Part model, mm, in its own coordinate system. Face numbers are marked on the shaded views. A direction names the side the tool comes from. Coordinates: 2 decimals unless noted, no trailing zeros. Loops run counter-clockwise (first coordinate to the right, second up) from the corner with the lowest first, then second, coordinate; pieces in that order, holes last. Notation, with made-up numbers: M 80,-28.75 L 96,-28.75 A8 ccw 96,-17.75 Z; hole C 26.25,72.5 d6. An arc over 180 degrees is marked long. Use a Markdown table: item, result. Add a question column.
1) Band-saw the part on D-D (x = 3). List the corners of the cut face in (y, z).
2) Band-saw the part on B-B (y = 1.75). List the corners of the cut face in (x, z), plus the area to 3 significant figures.
3) Tool access for the marked faces 4, 5 and 6: list every direction of +Z, -Z, +X, -X, +Y, -Y with a clear straight run to the whole face (end or side of a thin tool).
4) Band-saw the part on A-A (z = -3.5). List the corners of the cut face in (x, y), plus the area to 3 significant figures.
5) Wall check: probe 1 along Z at (x, y) = (2, 0.55); probe 2 along Z at (x, y) = (3, 2.4); probe 3 along X at (y, z) = (2.05, 3). Give the ranges that are in metal, low to high. Write a range as from..to.
6) Pull direction X, two halves, no side cores. Call the marked faces 1, 2 and 3: released by +X, released by -X, zero draft, split by the parting line, or undercut.
7) Pin check, flat tips, straight feed: pin 1 Ø10.5 at (x, z) = (0, 0) entering from +Y; pin 2 Ø0.9 at (x, y) = (17.5, 2) entering from +Z; pin 3 Ø0.9 at (y, z) = (2, -17) entering from -X; pin 4 Ø0.9 at (y, z) = (2, -20.5) entering from +X. Stop position of each tip, or through.
8) Band-saw the part on C-C (z = 3). List the corners of the cut face in (x, y).
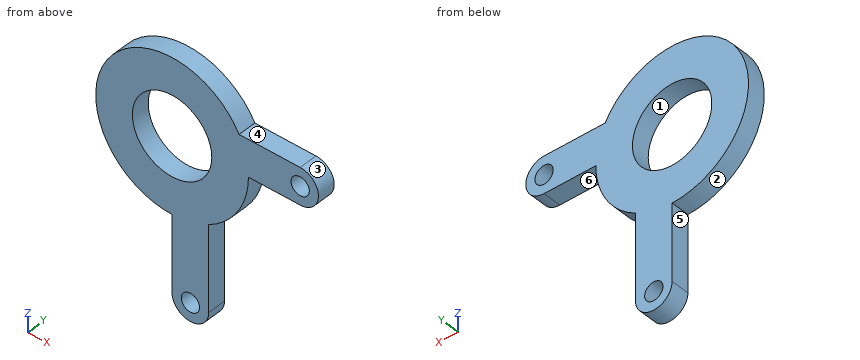
from build123d import *

# Parameters (mm, degrees)
SKETCH1_R           = 6.5
SKETCH1_R_2         = 1.5
BOSS_EXTRUDE1_DEPTH = 3


with BuildPart() as part:
    # Sketch1 → Boss-Extrude1 (new body)
    with BuildSketch(Plane(origin=(0, 0, 0), x_dir=(1, 0, 0), z_dir=(0, 1, 0))):
        with BuildLine():
            Line((0, 12.5), (0, 24.9658561))
            ThreePointArc((0, 24.9658561), (3, 27.9658561), (6, 24.9658561))
            Line((6, 24.9658561), (6, 10.9658561))
            ThreePointArc((6, 10.9658561), (10.752906584, 6.373774392), (12.5, 0))
            Line((12.5, 0), (20.9658561, 0))
            ThreePointArc((20.9658561, 0), (23.9658561, -3), (20.9658561, -6))
            Line((20.9658561, -6), (10.9658561, -6))
            ThreePointArc((10.9658561, -6), (-10.752906584, -6.373774392), (0, 12.5))
        make_face()
        Circle(SKETCH1_R, mode=Mode.SUBTRACT)
        with Locations((3, 24.9658561)):
            Circle(SKETCH1_R_2, mode=Mode.SUBTRACT)
        with Locations((20.9658561, -3)):
            Circle(SKETCH1_R_2, mode=Mode.SUBTRACT)
    extrude(amount=BOSS_EXTRUDE1_DEPTH)


solid = part.part
Entries:
| question | item | result |
|---|---|---|
| 1 | outline | M 0,-27.97 L 3,-27.97 L 3,-26.47 L 0,-26.47 Z; M 0,-23.47 L 3,-23.47 L 3,-5.77 L 0,-5.77 Z; M 0,5.77 L 3,5.77 L 3,12.13 L 0,12.13 Z |
| 2 | outline | M 0,-24.97 A3 ccw 6,-24.97 L 6,-10.97 A12.5 ccw 12.5,0 L 20.97,0 A3 ccw 20.97,6 L 10.97,6 A12.5 ccw long 0,-12.5 Z; hole C 0,0 d13; hole C 3,-24.97 d3; hole C 20.97,3 d3 |
| 2 | area | 504 mm2 |
| 3 | face 4 | +Z, +X, +Y, -Y |
| 3 | face 5 | -Z, -X, +Y, -Y |
| 3 | face 6 | -Z, +X, +Y, -Y |
| 4 | outline | M -12,0 L -5.48,0 L -5.48,3 L -12,3 Z; M 5.48,0 L 12,0 L 12,3 L 5.48,3 Z |
| 4 | area | 39.1 mm2 |
| 5 | probe 1 | -27.79..-26.08, -23.85..-6.18, 6.18..12.34 |
| 5 | probe 2 | -27.97..-26.47, -23.47..-5.77, 5.77..12.13 |
| 5 | probe 3 | -12.13..-5.77, 5.77..19.47, 22.47..23.97 |
| 6 | face 1 | undercut |
| 6 | face 2 | split by the parting line |
| 6 | face 3 | released by +X |
| 7 | pin 1 | through |
| 7 | pin 2 | z = 6 |
| 7 | pin 3 | x = 0 |
| 7 | pin 4 | x = 6 |
| 8 | outline | M -12.13,0 L -5.77,0 L -5.77,3 L -12.13,3 Z; M 5.77,0 L 19.47,0 L 19.47,3 L 5.77,3 Z; M 22.47,0 L 23.97,0 L 23.97,3 L 22.47,3 Z |
